The drawing under review shows one solid part. Ordinate dimensions are in mm from its lowest x, y, z. A direction names the side the tool comes from. Round coordinates to 2 decimals unless told otherwise and drop trailing zeros. Order: outer loops, then holes, each group sorted by start corner. A loop starts at its lowest first (then second) coordinate and runs counter-clockwise, first axis right, second up. Notation, with made-up numbers: (46, 55) -> (58, 55) arc R9 cw to (58, 61) -> close; hole circle Ø3 at (31, 62.5). An arc over 180 degrees is marked (long way). Use a Markdown table: item, result. Add a question column.
1) Consider section A-A (y = 10). State the section outline as (x, z) points.
2) Wall thickness on line 1 along X through (y, z) = (0.3, 6.3); line 2 along Z through (x, y) = (32.5, 0.6); line 3 along Y through (x, z) = (20, 11.55): over which ranges is each line inside the solid? List them lowest first. Write a range as [from, to].
3) Machinability: for the marked faces 1 and 2, which of the approach directions +Z, -Z, +X, -X, +Y, -Y give a long, thin tool a straight path to every point of the face, cutting with its end or side? Answer none if there is none.
4) Consider section D-D (x = 11.5). State the section outline as (y, z) points, plus the area to 3 significant figures.
5) Consider section C-C (x = 7.5). State the section outline as (y, z) points, plus the area to 3 significant figures.
6) Consider section B-B (z = 6.3). State the section outline as (x, y) points.
7) Clearance check with flat-ended pins moving along their axes: P1, Ø2.5, axis at x = 32.5, z = 6.3, coming from the +Y side; P2, Ø4, axis at x = 31, z = 3, coming from the +Y side; P3, Ø3.5, axis at x = 22, y = 9, coming from the -Z side. State where each tip first meets the part, or that it passes through.
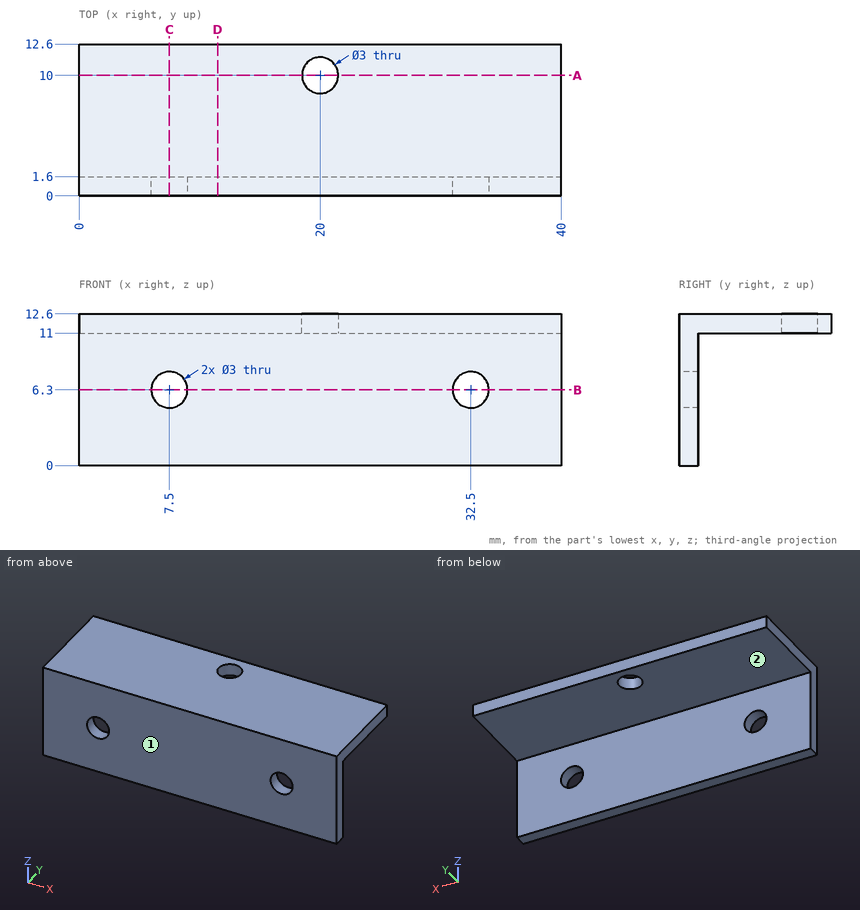
Results list:
| question | item | result |
|---|---|---|
| 1 | outline | (0, 11) -> (18.5, 11) -> (18.5, 12.6) -> (0, 12.6) -> close; (21.5, 11) -> (40, 11) -> (40, 12.6) -> (21.5, 12.6) -> close |
| 2 | line 1 | [0, 6], [9, 31], [34, 40] |
| 2 | line 2 | [0, 4.8], [7.8, 12.6] |
| 2 | line 3 | [0, 8.5], [11.5, 12.6] |
| 3 | face 1 | +Z, -Z, +X, -X, -Y |
| 3 | face 2 | -Z, +X, -X, +Y |
| 4 | outline | (0, 0) -> (1.6, 0) -> (1.6, 11) -> (12.6, 11) -> (12.6, 12.6) -> (0, 12.6) -> close |
| 4 | area | 37.8 mm2 |
| 5 | outline | (0, 0) -> (1.6, 0) -> (1.6, 4.8) -> (0, 4.8) -> close; (0, 7.8) -> (1.6, 7.8) -> (1.6, 11) -> (12.6, 11) -> (12.6, 12.6) -> (0, 12.6) -> close |
| 5 | area | 33.0 mm2 |
| 6 | outline | (0, 0) -> (6, 0) -> (6, 1.6) -> (0, 1.6) -> close; (9, 0) -> (31, 0) -> (31, 1.6) -> (9, 1.6) -> close; (34, 0) -> (40, 0) -> (40, 1.6) -> (34, 1.6) -> close |
| 7 | P1 | through |
| 7 | P2 | y = 1.6 |
| 7 | P3 | z = 11 |
